from build123d import *

# Parameters (mm, degrees)
F0_W     = 50
F0_H     = 16
F1_DEPTH = 3
F2_R     = 6
F2_R_2   = 3
F3_DEPTH = 8
F4_R     = 5


with BuildPart() as f1:
    # F0 (on Top) → F1 (new body)
    with BuildSketch(Plane.XY):
        Rectangle(F0_W, F0_H)
    extrude(amount=F1_DEPTH)

    # F2 (on Front) → F3 (join, symmetric)
    with BuildSketch(Plane.XZ):
        with Locations((0, 6)):
            Circle(F2_R)
        with Locations((0, 6)):
            Circle(F2_R_2, mode=Mode.SUBTRACT)
    extrude(amount=F3_DEPTH, both=True)

    # F4
    f4_edges = [f1.edges().sort_by_distance(p)[0] for p in [
        (-5.196152, 0, 3),
        (5.196152, 0, 3),
    ]]
    fillet(f4_edges, radius=F4_R)


solid = f1.part
The listing builds one solid part. Answer for the finished solid, in the listing's coordinates (mm). A direction names the side the tool comes from. Coordinates: 2 decimals unless noted, no trailing zeros. Loops run counter-clockwise (first coordinate to the right, second up) from the corner with the lowest first, then second, coordinate; pieces in that order, holes last.
1) Find the intervals of material crossed by L1, parallel to Z at x = 0, y = 0.75; L2, parallel to Z at x = -15, y = 1; L3, parallel to X at y = -4.25, z = 3.75, in increasing order.
2) Find section D-D on x = 13. Write down the section's boundary in (y, z).
3) Flat-ended cylindrical pins translate along their axes: pin 1 Ø1.5 at (y, z) = (1.5, 7.5) entering from -X; pin 2 Ø1.5 at (y, z) = (-2.5, 10.5) entering from -X; pin 3 Ø4 at (x, y) = (-11, -3.5) entering from +Z. Find the tip coordinate at first contact, or state that the pin passes through.
4) Find section C-C on z = 6. Write down the section's boundary in (x, y), then the cut area to 3 significant figures.
5) A tool of negligible diameter and unlimited length cuts with its end or side. For faces 1 (the face through (-18, 0, 3)), 2 (the face through (-25, 0, 1)), 3 (the face through (18, 0, 3)), from which of +Z, -Z, +X, -X, +Y, -Y can it reach the whole face along a straight path? Write none if from no direction.
6) Find section B-B on x = 0. Write down the section's boundary in (y, z), then the cut area to 3 significant figures.
7) Determine the mould class of faces 4 (the face through (-7.58, -0.11, 4.19)), 5 (the face through (-0.65, 0.11, 3.07)), 6 (the face through (25, 0, 1)), 7 (the face through (0, 0, 0)) for opening direction Z: pulls with the +Z half, pulls with the -Z half, needs draft (parallel to the pull), parting line crosses it, or undercut.
8) Find section A-A on y = 3. Write down the section's boundary in (x, z), then the cut area to 3 significant figures.
Values:
1. L1: z = 0 to 3, 9 to 12
1. L2: z = 0 to 3
1. L3: x = -8.18 to -1.98, 1.98 to 8.18
2. outline: (-8, 0) - (8, 0) - (8, 3) - (-8, 3) - close
3. pin 1: stops at x = -5.98
3. pin 2: stops at x = -4.68
3. pin 3: stops at z = 3.34
4. outline: (-6.23, -8) - (-3, -8) - (-3, 8) - (-6.23, 8) - close; (3, -8) - (6.23, -8) - (6.23, 8) - (3, 8) - close
4. area: 103 mm2
5. face 1: +Z, -X, +Y, -Y
5. face 2: +Z, -Z, -X, +Y, -Y
5. face 3: +Z, +X, +Y, -Y
6. outline: (-8, 0) - (8, 0) - (8, 3) - (-8, 3) - close; (-8, 9) - (8, 9) - (8, 12) - (-8, 12) - close
6. area: 96.0 mm2
7. face 4: pulls with the +Z half
7. face 5: undercut
7. face 6: needs draft
7. face 7: pulls with the -Z half
8. outline: (-25, 0) - (25, 0) - (25, 3) - (10.82, 3) arc R5 cw to (5.9, 7.09) arc R6 ccw to (-5.9, 7.09) arc R5 cw to (-10.82, 3) - (-25, 3) - close; hole circle Ø6 at (0, 6)
8. area: 224 mm2
